Work out the finished part from the listing and answer in its coordinate system (mm). A direction names the side the tool comes from. Coordinates: 2 decimals unless noted, no trailing zeros. Loops run counter-clockwise (first coordinate to the right, second up) from the corner with the lowest first, then second, coordinate; pieces in that order, holes last. Notation, with made-up numbers: M 11,-8 L 17,-8 A24 ccw 17,29 Z; hole C 63.5,75 d11. An arc over 180 degrees is marked long. Write each question's results on one line, items separated by ' | '.
```python
from build123d import *

# Parameters (mm, degrees)
SKETCH1_R           = 2.5
BOSS_EXTRUDE1_DEPTH = 200


with BuildPart() as part:
    # Sketch1 → Boss-Extrude1 (new body)
    with BuildSketch(Plane(origin=(0, 0, 0), x_dir=(1, 0, 0), z_dir=(0, 1, 0))):
        Polygon((-3.2, 10), (-3.2, 8.6), (-6.2, 8.6), (-6.2, 7.189949494), (-3, 3.989949494), (3, 3.989949494), (6.2, 7.189949494), (6.2, 8.6), (3.2, 8.6), (3.2, 10), (10, 10), (10, 3.2), (8.6, 3.2), (8.6, 6.2), (7.189949494, 6.2), (3.989949494, 3), (3.989949494, -3), (7.189949494, -6.2), (8.6, -6.2), (8.6, -3.2), (10, -3.2), (10, -10), (3.2, -10), (3.2, -8.6), (6.2, -8.6), (6.2, -7.189949494), (3, -3.989949494), (-3, -3.989949494), (-6.2, -7.189949494), (-6.2, -8.6), (-3.2, -8.6), (-3.2, -10), (-10, -10), (-10, -3.2), (-8.6, -3.2), (-8.6, -6.2), (-7.189949494, -6.2), (-3.989949494, -3), (-3.989949494, 3), (-7.189949494, 6.2), (-8.6, 6.2), (-8.6, 3.2), (-10, 3.2), (-10, 10), align=None)
        Circle(SKETCH1_R, mode=Mode.SUBTRACT)
    extrude(amount=BOSS_EXTRUDE1_DEPTH)


solid = part.part
```
1) Straight lines are drawn through the part: probe 1 along X at (y, z) = (95, 0); probe 2 along X at (y, z) = (146, -7.5). For each, find the intervals that lie inside material, in ascending order. Write a range as [from, to].
Check result:
probe 1: [-3.99, -2.5], [2.5, 3.99] | probe 2: [-10, -6.2], [6.2, 10]
2) Find section A-A, the plane z = 0. Give the vertices of the cut face in (x, y), and give its area (3 significant figures).
Check result:
outline: M -3.99,0 L -2.5,0 L -2.5,200 L -3.99,200 Z; M 2.5,0 L 3.99,0 L 3.99,200 L 2.5,200 Z | area: 596 mm^2
3) Which of the six approach directions +Z, -Z, +X, -X, +Y, -Y give full straight-line access (tool end or side, diameter ignored) to faces 1 (the face through (3.99, 99, 0)), 2 (the face through (-5.61, 98.6, 4.62)), 3 (the face through (-3.99, 99, 0)), 4 (the face through (0, 99, 3.99))?
Check result:
face 1: +X, +Y, -Y | face 2: +Y, -Y | face 3: -X, +Y, -Y | face 4: +Z, +Y, -Y
4) For a pull along Z with two mould halves and no side action, classify faces 5 (the face through (-10, 99, -7)), 6 (the face through (4.62, 98.6, 5.61)), 7 (the face through (-7, 99, -10)) as released by +Z, released by -Z, zero draft, split by the parting line, or undercut.
Check result:
face 5: zero draft | face 6: undercut | face 7: released by -Z
5) Find section B-B, the plane x = 0. Give the vertices of the cut face in (y, z), and give its area (3 significant figures).
Check result:
outline: M 0,-3.99 L 200,-3.99 L 200,-2.5 L 0,-2.5 Z; M 0,2.5 L 200,2.5 L 200,3.99 L 0,3.99 Z | area: 596 mm^2
